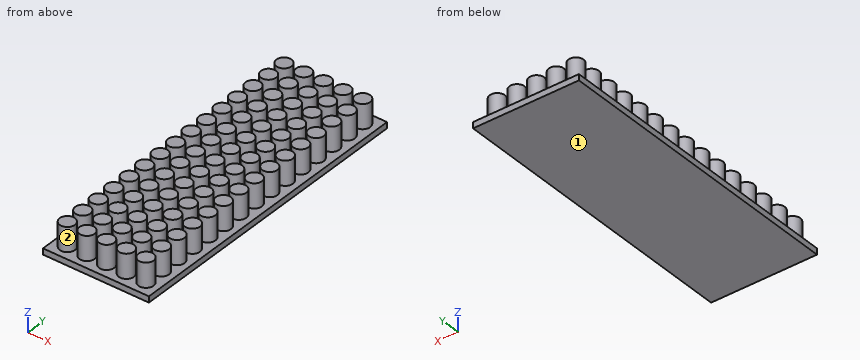
```python
from build123d import *

# Parameters (mm, degrees)
F0_W     = 17.5
F0_H     = 50
F0_R     = 1.25
F1_DEPTH = 1
F2_DEPTH = 5


with BuildPart() as f1:
    # F0 (on Top) → F1 (new body)
    with BuildSketch(Plane.XY):
        Rectangle(F0_W, F0_H)
        with Locations((-6.5, -22.75)):
            Circle(F0_R, mode=Mode.SUBTRACT)
        with Locations((-6.5, -19.5)):
            Circle(F0_R, mode=Mode.SUBTRACT)
        with Locations((-6.5, -16.25)):
            Circle(F0_R, mode=Mode.SUBTRACT)
        with Locations((-6.5, -13)):
            Circle(F0_R, mode=Mode.SUBTRACT)
        with Locations((-3.25, -22.75)):
            Circle(F0_R, mode=Mode.SUBTRACT)
        with Locations((-3.25, -19.5)):
            Circle(F0_R, mode=Mode.SUBTRACT)
        with Locations((-3.25, -16.25)):
            Circle(F0_R, mode=Mode.SUBTRACT)
        with Locations((-3.25, -13)):
            Circle(F0_R, mode=Mode.SUBTRACT)
        with Locations((-6.5, -9.75)):
            Circle(F0_R, mode=Mode.SUBTRACT)
        with Locations((-6.5, -6.5)):
            Circle(F0_R, mode=Mode.SUBTRACT)
        with Locations((-6.5, -3.25)):
            Circle(F0_R, mode=Mode.SUBTRACT)
        with Locations((-3.25, -9.75)):
            Circle(F0_R, mode=Mode.SUBTRACT)
        with Locations((-3.25, -6.5)):
            Circle(F0_R, mode=Mode.SUBTRACT)
        with Locations((-3.25, -3.25)):
            Circle(F0_R, mode=Mode.SUBTRACT)
        with Locations((0, -22.75)):
            Circle(F0_R, mode=Mode.SUBTRACT)
        with Locations((0, -19.5)):
            Circle(F0_R, mode=Mode.SUBTRACT)
        with Locations((3.25, -22.75)):
            Circle(F0_R, mode=Mode.SUBTRACT)
        with Locations((3.25, -19.5)):
            Circle(F0_R, mode=Mode.SUBTRACT)
        with Locations((0, -16.25)):
            Circle(F0_R, mode=Mode.SUBTRACT)
        with Locations((0, -13)):
            Circle(F0_R, mode=Mode.SUBTRACT)
        with Locations((3.25, -16.25)):
            Circle(F0_R, mode=Mode.SUBTRACT)
        with Locations((3.25, -13)):
            Circle(F0_R, mode=Mode.SUBTRACT)
        with Locations((6.5, -22.75)):
            Circle(F0_R, mode=Mode.SUBTRACT)
        with Locations((6.5, -19.5)):
            Circle(F0_R, mode=Mode.SUBTRACT)
        with Locations((6.5, -16.25)):
            Circle(F0_R, mode=Mode.SUBTRACT)
        with Locations((6.5, -13)):
            Circle(F0_R, mode=Mode.SUBTRACT)
        with Locations((0, -9.75)):
            Circle(F0_R, mode=Mode.SUBTRACT)
        with Locations((0, -6.5)):
            Circle(F0_R, mode=Mode.SUBTRACT)
        with Locations((3.25, -9.75)):
            Circle(F0_R, mode=Mode.SUBTRACT)
        with Locations((3.25, -6.5)):
            Circle(F0_R, mode=Mode.SUBTRACT)
        with Locations((0, -3.25)):
            Circle(F0_R, mode=Mode.SUBTRACT)
        with Locations((3.25, -3.25)):
            Circle(F0_R, mode=Mode.SUBTRACT)
        with Locations((6.5, -9.75)):
            Circle(F0_R, mode=Mode.SUBTRACT)
        with Locations((6.5, -6.5)):
            Circle(F0_R, mode=Mode.SUBTRACT)
        with Locations((6.5, -3.25)):
            Circle(F0_R, mode=Mode.SUBTRACT)
        with Locations((-6.5, 0)):
            Circle(F0_R, mode=Mode.SUBTRACT)
        with Locations((-6.5, 3.25)):
            Circle(F0_R, mode=Mode.SUBTRACT)
        with Locations((-6.5, 6.5)):
            Circle(F0_R, mode=Mode.SUBTRACT)
        with Locations((-6.5, 9.75)):
            Circle(F0_R, mode=Mode.SUBTRACT)
        with Locations((-3.25, 0)):
            Circle(F0_R, mode=Mode.SUBTRACT)
        with Locations((-3.25, 3.25)):
            Circle(F0_R, mode=Mode.SUBTRACT)
        with Locations((-3.25, 6.5)):
            Circle(F0_R, mode=Mode.SUBTRACT)
        with Locations((-3.25, 9.75)):
            Circle(F0_R, mode=Mode.SUBTRACT)
        with Locations((-6.5, 13)):
            Circle(F0_R, mode=Mode.SUBTRACT)
        with Locations((-6.5, 16.25)):
            Circle(F0_R, mode=Mode.SUBTRACT)
        with Locations((-6.5, 19.5)):
            Circle(F0_R, mode=Mode.SUBTRACT)
        with Locations((-6.5, 22.75)):
            Circle(F0_R, mode=Mode.SUBTRACT)
        with Locations((-3.25, 13)):
            Circle(F0_R, mode=Mode.SUBTRACT)
        with Locations((-3.25, 16.25)):
            Circle(F0_R, mode=Mode.SUBTRACT)
        with Locations((-3.25, 19.5)):
            Circle(F0_R, mode=Mode.SUBTRACT)
        with Locations((-3.25, 22.75)):
            Circle(F0_R, mode=Mode.SUBTRACT)
        Circle(F0_R, mode=Mode.SUBTRACT)
        with Locations((0, 3.25)):
            Circle(F0_R, mode=Mode.SUBTRACT)
        with Locations((3.25, 0)):
            Circle(F0_R, mode=Mode.SUBTRACT)
        with Locations((3.25, 3.25)):
            Circle(F0_R, mode=Mode.SUBTRACT)
        with Locations((0, 6.5)):
            Circle(F0_R, mode=Mode.SUBTRACT)
        with Locations((0, 9.75)):
            Circle(F0_R, mode=Mode.SUBTRACT)
        with Locations((3.25, 6.5)):
            Circle(F0_R, mode=Mode.SUBTRACT)
        with Locations((3.25, 9.75)):
            Circle(F0_R, mode=Mode.SUBTRACT)
        with Locations((6.5, 0)):
            Circle(F0_R, mode=Mode.SUBTRACT)
        with Locations((6.5, 3.25)):
            Circle(F0_R, mode=Mode.SUBTRACT)
        with Locations((6.5, 6.5)):
            Circle(F0_R, mode=Mode.SUBTRACT)
        with Locations((6.5, 9.75)):
            Circle(F0_R, mode=Mode.SUBTRACT)
        with Locations((0, 13)):
            Circle(F0_R, mode=Mode.SUBTRACT)
        with Locations((0, 16.25)):
            Circle(F0_R, mode=Mode.SUBTRACT)
        with Locations((3.25, 13)):
            Circle(F0_R, mode=Mode.SUBTRACT)
        with Locations((3.25, 16.25)):
            Circle(F0_R, mode=Mode.SUBTRACT)
        with Locations((0, 19.5)):
            Circle(F0_R, mode=Mode.SUBTRACT)
        with Locations((0, 22.75)):
            Circle(F0_R, mode=Mode.SUBTRACT)
        with Locations((3.25, 19.5)):
            Circle(F0_R, mode=Mode.SUBTRACT)
        with Locations((3.25, 22.75)):
            Circle(F0_R, mode=Mode.SUBTRACT)
        with Locations((6.5, 13)):
            Circle(F0_R, mode=Mode.SUBTRACT)
        with Locations((6.5, 16.25)):
            Circle(F0_R, mode=Mode.SUBTRACT)
        with Locations((6.5, 19.5)):
            Circle(F0_R, mode=Mode.SUBTRACT)
        with Locations((6.5, 22.75)):
            Circle(F0_R, mode=Mode.SUBTRACT)
        with Locations((3.25, 0)):
            Circle(F0_R)
        with Locations((6.5, 0)):
            Circle(F0_R)
    extrude(amount=F1_DEPTH)

    # F0 (on Top) → F2 (join)
    with BuildSketch(Plane.XY):
        Circle(F0_R)
        with Locations((0, 3.25)):
            Circle(F0_R)
        with Locations((0, 6.5)):
            Circle(F0_R)
        with Locations((0, 9.75)):
            Circle(F0_R)
        with Locations((0, 13)):
            Circle(F0_R)
        with Locations((0, 16.25)):
            Circle(F0_R)
        with Locations((0, 19.5)):
            Circle(F0_R)
        with Locations((0, 22.75)):
            Circle(F0_R)
        with Locations((3.25, 0)):
            Circle(F0_R)
        with Locations((3.25, 3.25)):
            Circle(F0_R)
        with Locations((3.25, 6.5)):
            Circle(F0_R)
        with Locations((3.25, 9.75)):
            Circle(F0_R)
        with Locations((3.25, 13)):
            Circle(F0_R)
        with Locations((3.25, 16.25)):
            Circle(F0_R)
        with Locations((3.25, 19.5)):
            Circle(F0_R)
        with Locations((3.25, 22.75)):
            Circle(F0_R)
        with Locations((6.5, 0)):
            Circle(F0_R)
        with Locations((6.5, 3.25)):
            Circle(F0_R)
        with Locations((6.5, 6.5)):
            Circle(F0_R)
        with Locations((6.5, 9.75)):
            Circle(F0_R)
        with Locations((6.5, 13)):
            Circle(F0_R)
        with Locations((6.5, 16.25)):
            Circle(F0_R)
        with Locations((6.5, 19.5)):
            Circle(F0_R)
        with Locations((6.5, 22.75)):
            Circle(F0_R)
        with Locations((-3.25, 19.5)):
            Circle(F0_R)
        with Locations((-6.5, 9.75)):
            Circle(F0_R)
        with Locations((-6.5, 6.5)):
            Circle(F0_R)
        with Locations((-6.5, 16.25)):
            Circle(F0_R)
        with Locations((-6.5, 3.25)):
            Circle(F0_R)
        with Locations((-6.5, 22.75)):
            Circle(F0_R)
        with Locations((-6.5, 13)):
            Circle(F0_R)
        with Locations((-3.25, 13)):
            Circle(F0_R)
        with Locations((-3.25, 9.75)):
            Circle(F0_R)
        with Locations((-3.25, 6.5)):
            Circle(F0_R)
        with Locations((-3.25, 16.25)):
            Circle(F0_R)
        with Locations((-3.25, 3.25)):
            Circle(F0_R)
        with Locations((-3.25, 22.75)):
            Circle(F0_R)
        with Locations((-6.5, 19.5)):
            Circle(F0_R)
        with Locations((-3.25, -22.75)):
            Circle(F0_R)
        with Locations((-3.25, -19.5)):
            Circle(F0_R)
        with Locations((-3.25, -9.75)):
            Circle(F0_R)
        with Locations((-6.5, -16.25)):
            Circle(F0_R)
        with Locations((-3.25, -6.5)):
            Circle(F0_R)
        with Locations((-3.25, -16.25)):
            Circle(F0_R)
        with Locations((-3.25, -3.25)):
            Circle(F0_R)
        with Locations((-6.5, -9.75)):
            Circle(F0_R)
        with Locations((-6.5, -19.5)):
            Circle(F0_R)
        with Locations((-6.5, -22.75)):
            Circle(F0_R)
        with Locations((-6.5, -13)):
            Circle(F0_R)
        with Locations((-6.5, -6.5)):
            Circle(F0_R)
        with Locations((-6.5, -3.25)):
            Circle(F0_R)
        with Locations((-3.25, -13)):
            Circle(F0_R)
        with Locations((3.25, -13)):
            Circle(F0_R)
        with Locations((3.25, -9.75)):
            Circle(F0_R)
        with Locations((6.5, -16.25)):
            Circle(F0_R)
        with Locations((3.25, -6.5)):
            Circle(F0_R)
        with Locations((3.25, -3.25)):
            Circle(F0_R)
        with Locations((3.25, -22.75)):
            Circle(F0_R)
        with Locations((3.25, -19.5)):
            Circle(F0_R)
        with Locations((6.5, -6.5)):
            Circle(F0_R)
        with Locations((6.5, -19.5)):
            Circle(F0_R)
        with Locations((6.5, -13)):
            Circle(F0_R)
        with Locations((6.5, -3.25)):
            Circle(F0_R)
        with Locations((6.5, -22.75)):
            Circle(F0_R)
        with Locations((3.25, -16.25)):
            Circle(F0_R)
        with Locations((6.5, -9.75)):
            Circle(F0_R)
        with Locations((0, -6.5)):
            Circle(F0_R)
        with Locations((0, -9.75)):
            Circle(F0_R)
        with Locations((0, -22.75)):
            Circle(F0_R)
        with Locations((0, -19.5)):
            Circle(F0_R)
        with Locations((0, -16.25)):
            Circle(F0_R)
        with Locations((0, -13)):
            Circle(F0_R)
        with Locations((0, -3.25)):
            Circle(F0_R)
        with Locations((-6.5, 0)):
            Circle(F0_R)
        with Locations((-3.25, 0)):
            Circle(F0_R)
    extrude(amount=F2_DEPTH)


solid = f1.part
```
Geometry: final body of the model. Coordinates: model frame, mm. Face numbers are marked on the shaded views. Round coordinates to 2 decimals unless told otherwise and drop trailing zeros. Order: outer loops, then holes, each group sorted by start corner. A loop starts at its lowest first (then second) coordinate and runs counter-clockwise, first axis right, second up. Notation, with made-up numbers: M 7.5,-12 L 58.5,-12 A21 cw 58.5,3 Z; hole C 11,76 d2. An arc over 180 degrees is marked long. One line per item, written item: value.
(1) Pull-direction query (X, two-part tool) for the marked faces 1 and 2; classes: pulls with the +X half, pulls with the -X half, needs draft (parallel to the pull), parting line crosses it, or undercut.
Result sheet:
face 1: needs draft
face 2: undercut
(2) Cut plane C-C (y = -12.5). Return the cut outline in (x, z), and give its area (3 significant figures).
Result sheet:
outline: M -8.75,0 L 8.75,0 L 8.75,1 L 7.65,1 L 7.65,5 L 5.35,5 L 5.35,1 L 4.4,1 L 4.4,5 L 2.1,5 L 2.1,1 L 1.15,1 L 1.15,5 L -1.15,5 L -1.15,1 L -2.1,1 L -2.1,5 L -4.4,5 L -4.4,1 L -5.35,1 L -5.35,5 L -7.65,5 L -7.65,1 L -8.75,1 Z
area: 63.3 mm2
(3) Cut plane A-A (y = 13). Return the cut outline in (x, z), and give its area (3 significant figures).
Result sheet:
outline: M -8.75,0 L 8.75,0 L 8.75,1 L 7.75,1 L 7.75,5 L 5.25,5 L 5.25,1 L 4.5,1 L 4.5,5 L 2,5 L 2,1 L 1.25,1 L 1.25,5 L -1.25,5 L -1.25,1 L -2,1 L -2,5 L -4.5,5 L -4.5,1 L -5.25,1 L -5.25,5 L -7.75,5 L -7.75,1 L -8.75,1 Z
area: 67.5 mm2
(4) Cut plane B-B (z = 3.05). Give the number of separate pieces and of enclosed holes in the cut face, and give its area (3 significant figures).
Result sheet:
separate pieces: 75
enclosed holes: 0
area: 368 mm2
(5) Line query: probe 1 along X at (y, z) = (-13.5, 4.7); probe 2 along X at (y, z) = (3, 4.85); probe 3 along Z at (x, y) = (1.5, -16). Output: solid intervals per line, ascending. Write a range as [from, to].
Result sheet:
probe 1: [-7.65, -5.35], [-4.4, -2.1], [-1.15, 1.15], [2.1, 4.4], [5.35, 7.65]
probe 2: [-7.72, -5.28], [-4.47, -2.03], [-1.22, 1.22], [2.03, 4.47], [5.28, 7.72]
probe 3: [0, 1]
